Here's how the part is built. I have some questions about the finished solid (model axes, mm). Face numbers are marked on the shaded views. Round coordinates to 2 decimals unless told otherwise and drop trailing zeros. Order: outer loops, then holes, each group sorted by start corner. A loop starts at its lowest first (then second) coordinate and runs counter-clockwise, first axis right, second up. Notation, with made-up numbers: (37, 42) - (79, 42) arc R20 ccw to (79, 76) - close; hole circle Ø5 at (54, -17). An arc over 180 degrees is marked (long way). Answer as a JSON object with one key per item and string values.
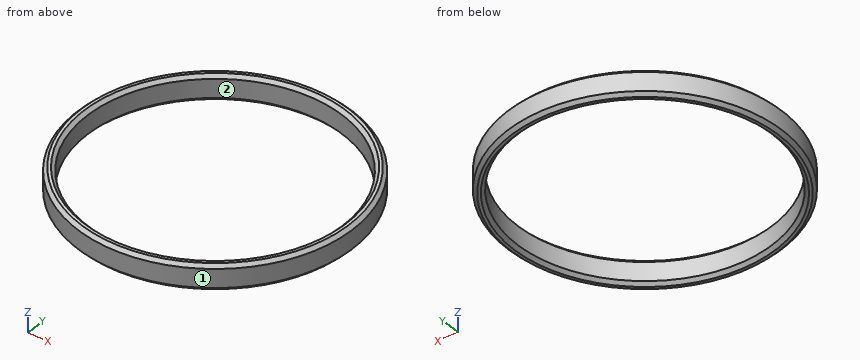
```python
from build123d import *

# Parameters (mm, degrees)
F0_R     = 16.25
F1_DEPTH = 3
F2_R     = 15.1
F3_DEPTH = 3.001
F4_SIZE  = 0.4
F5_SIZE  = 0.4


with BuildPart() as f1:
    # F0 (on Top) → F1 (new body)
    with BuildSketch(Plane.XY):
        Circle(F0_R)
    extrude(amount=F1_DEPTH)

    # F2 (on face) → F3 (cut, through all)
    with BuildSketch(Plane.XY.offset(3)):
        Circle(F2_R)
    extrude(amount=-F3_DEPTH, mode=Mode.SUBTRACT)

    # F4
    f4_edges = [f1.edges().sort_by_distance(p)[0] for p in [
        (-15.1, 0, 3),
        (-15.1, 0, 0),
    ]]
    chamfer(f4_edges, length=F4_SIZE)

    # F5
    f5_edges = [f1.edges().sort_by_distance(p)[0] for p in [
        (-16.25, 0, 0),
        (-16.25, 0, 3),
    ]]
    chamfer(f5_edges, length=F5_SIZE)


solid = f1.part
```
1. Thinking about a two-plate mould opening in X: for the marked faces 1 and 2, which applies, pulls with the +X half, pulls with the -X half, needs draft (parallel to the pull), parting line crosses it, or undercut?
Responses:
{"face 1": "parting line crosses it", "face 2": "undercut"}
2. Imagine slicing it at C-C (z = 1.4). List the corners of the cut face in (x, y) for me.
Responses:
{"outline": "circle Ø32.5 at (0, 0); hole circle Ø30.2 at (0, 0)"}
3. Imagine slicing it at A-A (y = 0). List the corners of the cut face in (x, z) for me.
Responses:
{"outline": "(-16.25, 0.4) - (-15.85, 0) - (-15.5, 0) - (-15.1, 0.4) - (-15.1, 2.6) - (-15.5, 3) - (-15.85, 3) - (-16.25, 2.6) - close; (15.1, 0.4) - (15.5, 0) - (15.85, 0) - (16.25, 0.4) - (16.25, 2.6) - (15.85, 3) - (15.5, 3) - (15.1, 2.6) - close"}
4. For P1, Ø6, axis at x = -5, y = 9.5, coming from the +Z side; P2, Ø1.5, axis at y = 11, z = 1.5, coming from the +X side; P3, Ø1.5, axis at x = 3.5, z = 1.5, coming from the -Y side, each with a flat end and sliding along its axis, tell me the tip position at first contact or that it passes through.
Responses:
{"P1": "through", "P2": "x = 12.61", "P3": "y = -16.02"}
5. If I drill on L1, parallel to Y at x = 0, z = 1.9; L2, parallel to Y at x = -9, z = 2.8; L3, parallel to X at y = 12, z = 2.65, over which ranges is the centre line in solid material (lowest first)? Write a range as [from, to].
Responses:
{"L1": "[-16.25, -15.1], [15.1, 16.25]", "L2": "[-13.29, -12.37], [12.37, 13.29]", "L3": "[-10.88, -9.25], [9.25, 10.88]"}
